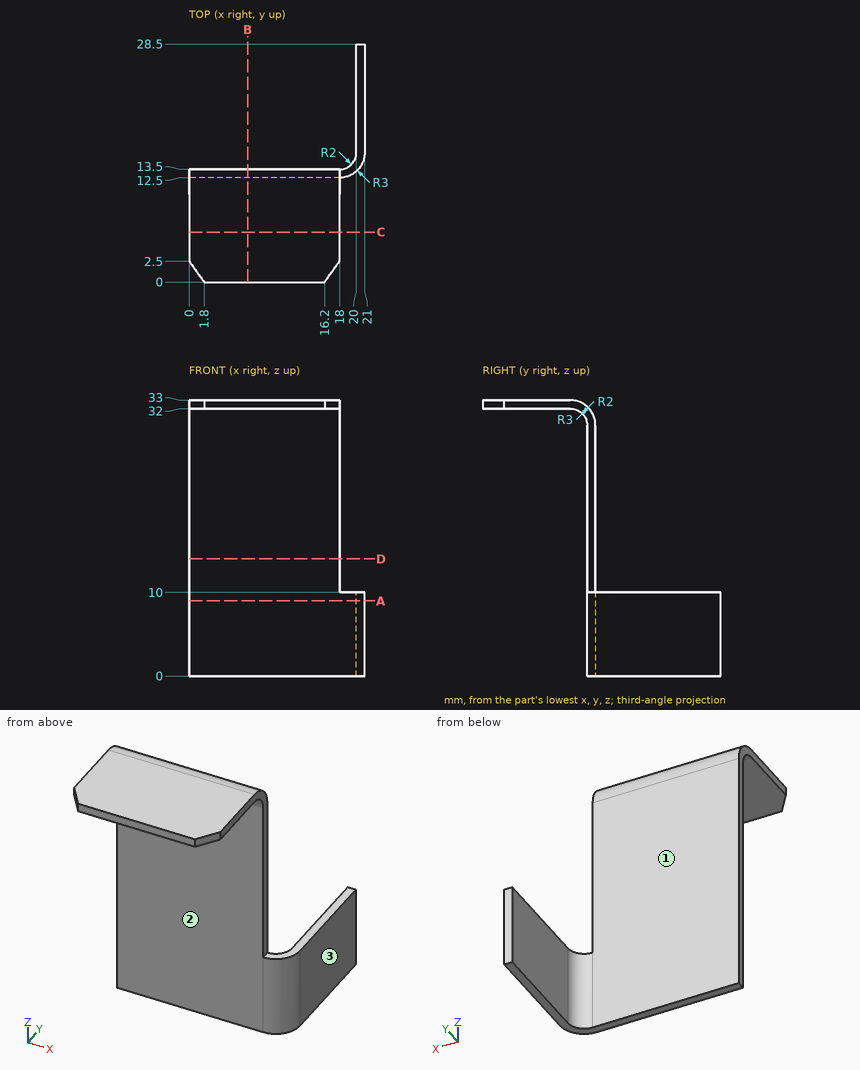
Part print with two shaded views. Sizes in mm from the minimum x, y, z corner. A direction names the side the tool comes from. Round coordinates to 2 decimals unless told otherwise and drop trailing zeros. Write each loop counter-clockwise with the first axis right and the second up, starting at its lowest first coordinate (ties: lowest second). Pieces come first, ordered by that corner, then holes. Notation, with made-up numbers: M 16.25,35.5 L 71.25,35.5 A25 ccw 71.25,72.5 Z; hole C -17.5,6 d8. An arc over 180 degrees is marked long. Put each result on its own line as item: value. Start each with the question number.
1) Saw through at D-D, the plane z = 14. Write the cut outline in (x, y).
2) Drill centre lines: probe 1 along Y at (x, z) = (13.25, 26.5); probe 2 along X at (y, z) = (15.5, 5); probe 3 along Z at (x, y) = (17, 4). Where is each one in solid material? Low to high. Write a range as [from, to].
3) Saw through at B-B, the plane x = 7. Write the cut outline in (y, z).
4) Saw through at C-C, the plane y = 6. Write the cut outline in (x, z).
5) 3-axis set-ups, long thin cutter, end or side, ignore diameter. For the marked faces 1, 2 and 3: which of +Z, -Z, +X, -X, +Y, -Y reach the whole face in a straight line?
6) Saw through at A-A, the plane z = 9. Write the cut outline in (x, y), and give its area (3 significant figures).
7) Pin check, flat tips, straight feed: pin 1 Ø3 at (x, y) = (11.5, 3) entering from -Z; pin 2 Ø6 at (x, z) = (13.5, 18.5) entering from +Y; pin 3 Ø6 at (x, z) = (3, 15) entering from -Y; pin 4 Ø10 at (y, z) = (20, 11) entering from +X. Stop position of each tip, or through.
Resolved:
1. outline: M 0,12.5 L 18,12.5 L 18,13.5 L 0,13.5 Z
2. probe 1: [12.5, 13.5]
2. probe 2: [20, 21]
2. probe 3: [32, 33]
3. outline: M 0,32 L 10.5,32 A2 cw 12.5,30 L 12.5,0 L 13.5,0 L 13.5,30 A3 ccw 10.5,33 L 0,33 Z
4. outline: M 0,32 L 18,32 L 18,33 L 0,33 Z
5. face 1: +Z, -Z, -X, +Y
5. face 2: -Z, +X, -X, -Y
5. face 3: +Z, -Z, +X, +Y, -Y
6. outline: M 0,12.5 L 18,12.5 A3 ccw 21,15.5 L 21,28.5 L 20,28.5 L 20,15.5 A2 cw 18,13.5 L 0,13.5 Z
6. area: 34.9 mm²
7. pin 1: z = 32
7. pin 2: y = 13.5
7. pin 3: y = 12.5
7. pin 4: x = 21
